```python
from build123d import *

# Parameters (mm, degrees)
SKETCH_1_R          = 8.075
EXTRUDE_1_DEPTH     = 7
EXTRUDE_START       = -2
SKETCH_2_R          = 8.075
SKETCH_2_R_2        = 6.575
EXTRUDE_2_DEPTH     = 2
SKETCH_3_R          = 4
EXTRUDE_3_DEPTH     = 10
SKETCH_4_R          = 5
SKETCH_4_R_2        = 4
EXTRUDE_4_DEPTH     = 3
CHAMFER_1_SIZE      = 0.5
CUT_EXTRUDE_1_DEPTH = 7
CUT_EXTRUDE_2_DEPTH = 5
CUT_EXTRUDE_START   = -2
SKETCH_8_R          = 4
CUT_EXTRUDE_3_DEPTH = 2
FILLET_1_R          = 0.5
SKETCH_9_R          = 2.2
CUT_EXTRUDE_4_DEPTH = 10
EXTRUDE_START_2     = 3
SKETCH_10_R         = 10.075
SKETCH_10_R_2       = 8.075
EXTRUDE_5_DEPTH     = 3
EXTRUDE_6_DEPTH     = 2
EXTRUDE_START_3     = 5
EXTRUDE_7_DEPTH     = 5


with BuildPart() as part:
    # 草图1 → 凸台-拉伸1 (new body)
    with BuildSketch(Plane.XY):
        with BuildLine():
            ThreePointArc((0.395882675, 11.067922204), (-11.074999998, -0.000217919), (0.396318234, -11.067906616))
            Line((0.396318234, -11.067906616), (114, -7))
            ThreePointArc((114, -7), (120.998881523, -0.125129643), (114.250219298, 6.995526449))
            Line((114.250219298, 6.995526449), (0.395882675, 11.067922204))
        make_face()
        Circle(SKETCH_1_R, mode=Mode.SUBTRACT)
    extrude(amount=EXTRUDE_1_DEPTH)

    # 草图2 → 凸台-拉伸2 (add)
    with BuildSketch(Plane.XY.offset(7).offset(EXTRUDE_START)):
        Circle(SKETCH_2_R)
        Circle(SKETCH_2_R_2, mode=Mode.SUBTRACT)
    extrude(amount=EXTRUDE_2_DEPTH)

    # 草图3 → 凸台-拉伸3 (add)
    with BuildSketch(Plane(origin=(0, 0, 0), x_dir=(-1, 0, 0), z_dir=(0, 0, -1))):
        with Locations((-114, 0)):
            Circle(SKETCH_3_R)
    extrude(amount=EXTRUDE_3_DEPTH)

    # 草图4 → 凸台-拉伸4 (add)
    with BuildSketch(Plane(origin=(0, 0, 0), x_dir=(-1, 0, 0), z_dir=(0, 0, -1))):
        with Locations(Location((-114, 0, 0), (0, 0, 180))):
            Circle(SKETCH_4_R)
        with Locations((-114, 0)):
            Circle(SKETCH_4_R_2, mode=Mode.SUBTRACT)
    extrude(amount=EXTRUDE_4_DEPTH)

    # 倒角1
    chamfer_1_edges = [part.edges().sort_by_distance(p)[0] for p in [
        (-6.575, 0, 5),
        (-6.575, 0, 7),
        (118, 0, -10),
        (109, 0, -3),
    ]]
    chamfer(chamfer_1_edges, length=CHAMFER_1_SIZE)

    # 草图5 → 切除-拉伸1 (cut)
    with BuildSketch(Plane(origin=(0, 0, 0), x_dir=(-1, 0, 0), z_dir=(0, 0, -1))):
        with BuildLine():
            ThreePointArc((-12.757234161, -4.640431182), (-13.574999998, 0.000234775), (-12.757073645, 4.640872443))
            Line((-12.757073645, 4.640872443), (-104.114755838, 1.510611753))
            ThreePointArc((-104.114755838, 1.510611753), (-104.028730231, 0.75748214), (-104, 0))
            ThreePointArc((-104, 0), (-104.028593207, -0.755676237), (-104.114209315, -1.507031033))
            Line((-104.114209315, -1.507031033), (-12.757234161, -4.640431182))
        make_face()
    extrude(amount=-CUT_EXTRUDE_1_DEPTH, mode=Mode.SUBTRACT)

    # 草图6 → 切除-拉伸2 (cut)
    with BuildSketch(Plane(origin=(0, 0, 0), x_dir=(-1, 0, 0), z_dir=(0, 0, -1))):
        Polygon((-104.114209315, -1.507031033), (-12.757234161, -4.640431182), (-12.860068961, -7.638668165), (-104.217044114, -4.505268015), align=None)
        Polygon((-12.757073645, 4.640872443), (-104.114755838, 1.510611753), (-104.217486931, 4.508852291), (-12.859804737, 7.63911298), align=None)
    extrude(amount=-CUT_EXTRUDE_2_DEPTH, mode=Mode.SUBTRACT)

    # 草图8 → 切除-拉伸3 (cut)
    with BuildSketch(Plane(origin=(0, 0, -10), x_dir=(-1, 0, 0), z_dir=(0, 0, -1)).offset(CUT_EXTRUDE_START)):
        with Locations((-114, 0)):
            Circle(SKETCH_8_R)
    extrude(amount=CUT_EXTRUDE_3_DEPTH, mode=Mode.SUBTRACT)

    # 圆角1
    fillet_1_edges = [part.edges().sort_by_distance(p)[0] for p in [
        (118, 0, -8),
    ]]
    fillet(fillet_1_edges, radius=FILLET_1_R)

    # 草图9 → 切除-拉伸4 (cut)
    with BuildSketch(Plane(origin=(0, 0, -8), x_dir=(-1, 0, 0), z_dir=(0, 0, -1))):
        with Locations((-114, 0)):
            Circle(SKETCH_9_R)
    extrude(amount=-CUT_EXTRUDE_4_DEPTH, mode=Mode.SUBTRACT)

    # 草图10 → 凸台-拉伸5 (add)
    with BuildSketch(Plane(origin=(0, 0, 0), x_dir=(-1, 0, 0), z_dir=(0, 0, -1)).offset(EXTRUDE_START_2)):
        with Locations(Location((0, 0, 0), (0, 0, 180))):
            Circle(SKETCH_10_R)
        Circle(SKETCH_10_R_2, mode=Mode.SUBTRACT)
    extrude(amount=-EXTRUDE_5_DEPTH)

    # 切除-旋转2: read off the stored shape, not the designer's step
    # 切除-旋转2: loft between two sections, ruled curve by curve
    cut_revolve_2_from = [
        Edge.make_three_point_arc((8.65, 0, -1.2), (0, 8.65, -1.2), (-8.65, 0, -1.2)),
        Edge.make_three_point_arc((-8.65, 0, -1.2), (0, -8.65, -1.2), (8.65, 0, -1.2)),
    ]
    cut_revolve_2_to = [
        Edge.make_three_point_arc((8.65, 0, 0), (0, 8.65, 0), (-8.65, 0, 0)),
        Edge.make_three_point_arc((-8.65, 0, 0), (0, -8.65, 0), (8.65, 0, 0)),
    ]
    cut_revolve_2 = Solid(Shell([*[Face.make_surface_from_curves(cut_revolve_2_from[k], cut_revolve_2_to[k]) for k in range(2)], Face(Wire(cut_revolve_2_from)), Face(Wire(cut_revolve_2_to))]))
    add(cut_revolve_2, mode=Mode.SUBTRACT)

    # 草图12 → 凸台-拉伸6 (add)
    with BuildSketch(Plane.XY.offset(7).offset(EXTRUDE_START)):
        with BuildLine():
            Line((104.114209315, -1.507031033), (12.757234161, -4.640431182))
            ThreePointArc((12.757234161, -4.640431182), (13.574999998, 0.000234775), (12.757073645, 4.640872443))
            Line((12.757073645, 4.640872443), (104.114755838, 1.510611753))
            ThreePointArc((104.114755838, 1.510611753), (104.000000164, 0.001811094), (104.114209315, -1.507031033))
        make_face()
    extrude(amount=EXTRUDE_6_DEPTH)

    # 草图13 → 凸台-拉伸7 (add)
    with BuildSketch(Plane(origin=(0, 0, 5), x_dir=(-1, 0, 0), z_dir=(0, 0, -1)).offset(EXTRUDE_START_3)):
        with BuildLine():
            Line((-104.114209315, -1.507031033), (-104.217044114, -4.505268015))
            Line((-104.217044114, -4.505268015), (-12.860068961, -7.638668165))
            Line((-12.860068961, -7.638668165), (-12.757234161, -4.640431182))
            ThreePointArc((-12.757234161, -4.640431182), (-13.574999998, 0.000234775), (-12.757073645, 4.640872443))
            Line((-12.757073645, 4.640872443), (-12.859804737, 7.63911298))
            Line((-12.859804737, 7.63911298), (-104.217486931, 4.508852291))
            Line((-104.217486931, 4.508852291), (-104.114755838, 1.510611753))
            ThreePointArc((-104.114755838, 1.510611753), (-104.000000164, 0.001811094), (-104.114209315, -1.507031033))
        make_face()
    extrude(amount=-EXTRUDE_7_DEPTH)


solid = part.part
```
Geometry check sheet. Reference: the model listing, model coordinates, mm. A direction names the side the tool comes from. Round coordinates to 2 decimals unless told otherwise and drop trailing zeros. Order: outer loops, then holes, each group sorted by start corner. A loop starts at its lowest first (then second) coordinate and runs counter-clockwise, first axis right, second up. Notation, with made-up numbers: (38, 48.25) -> (76, 48.25) arc R14 ccw to (76, 67.25) -> close; hole circle Ø5 at (4, 40). An arc over 180 degrees is marked (long way). Return JSON: item names as keys, results as strings. Group by question number.
Q1. Gauge pin test, flat ends, axial feed: pin 1 (10 mm diameter, centred on x = -1, y = -3.5, fed in from -Z); pin 2 (8 mm diameter, centred on y = 7.5, z = -1, fed in from -X); pin 3 (11 mm diameter, centred on x = 33, y = -3.5, fed in from -Z). Record the tip position at first contact, or that the pin passes through.
Q2. Material ranges on probe 1 along Y at (x, z) = (0, -2.6) (3 decimals); probe 2 along Z at (x, y) = (0.5, -8.25); probe 3 along Y at (x, z) = (0, 5.95) (3 decimals), recorded low to high. Write a range as from..to.
Q3. Tool access check on faces 4 (the flat face through (-8, -3, -3)), 5 (the cylindrical face through (116.198, 0.097, -3.07)), 6 (the flat face through (6, -6, -1.2)). Record the directions out of +Z, -Z, +X, -X, +Y, -Y that give a thin tool (end or side, any length) a straight path to the whole face; none if there is none.
Q4. Section check A-A, the plane z = -4.5. Record the boundary of the cut face in (x, y), plus the area to 3 significant figures.
Q5. Release check for a two-part mould opening along Y. For faces 1 (the cylindrical face through (118.619, 1.915, -1.232)), 2 (the cylindrical face through (1.751, -7.883, -2.113)), 3 (the flat face through (56, 0, 0)) record: released by +Y, released by -Y, zero draft, split by the parting line, or undercut.
Q6. Section check B-B, the plane x = 105. Record the boundary of the cut face in (y, z).
Numbers:
{
 "1": {"pin 1": "z = -3", "pin 2": "x = -10.46", "pin 3": "z = 0"},
 "2": {"probe 1": "-10.075..-8.075, 8.075..10.075", "probe 2": "-3..-1.2, 0..7", "probe 3": "-11.075..-6.575, 6.575..11.075"},
 "3": {"face 4": "-Z, -X, +Y, -Y", "face 5": "-Z", "face 6": "none"},
 "4": {"outline": "circle Ø8 at (114, 0); hole circle Ø4.4 at (114, 0)", "area": "35.1 mm^2"},
 "5": {"face 1": "split by the parting line", "face 2": "undercut", "face 3": "zero draft"},
 "6": {"outline": "(-7.32, 0) -> (7.33, 0) -> (7.33, 7) -> (-7.32, 7) -> close"}
}
